Build history of the part. All positions in model axes, mm. Round coordinates to 2 decimals unless told otherwise and drop trailing zeros. Write each loop counter-clockwise with the first axis right and the second up, starting at its lowest first coordinate (ties: lowest second). Pieces come first, ordered by that corner, then holes. Notation, with made-up numbers: (10.25, 39.5) - (14.25, 39.5) arc R22 cw to (14.25, 57.5) - close; hole circle Ø11 at (-8, -35.5). An arc over 180 degrees is marked (long way). Write each question's results on one line, items separated by ' | '.
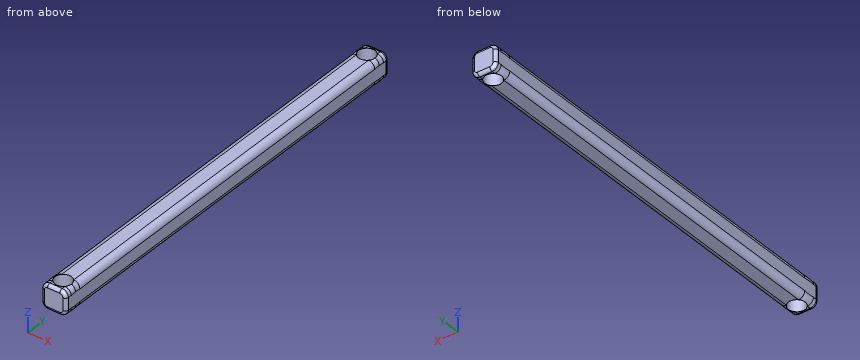
Autodesk Inventor part; units mm, degrees
ref_plane "YZ Plane" through (0, 0, 0) normal (1, 0, 0) x (0, 1, 0)
ref_plane "XZ Plane" through (0, 0, 0) normal (0, 1, 0) x (-1, 0, 0)
ref_plane "XY Plane" through (0, 0, 0) normal (0, 0, 1) x (1, 0, 0)
sketch "Sketch1" plane through (0, 0, 0) normal (0, 1, 0) x (-1, 0, 0)
  line L0 (-3.175, -3.175) -> (3.175, -3.175)
  line L1 (3.175, -3.175) -> (3.175, 3.175)
  line L2 (3.175, 3.175) -> (-3.175, 3.175)
  line L3 (-3.175, 3.175) -> (-3.175, -3.175)
  line L4 (-3.175, -3.175) -> (3.175, 3.175) construction
  line L5 (3.175, -3.175) -> (-3.175, 3.175) construction
  point P0 (0, 0)
  dimension "d0" = 6.35
  dimension "d1" = 6.35
extrude "Extrusion1" add sketch "Sketch1" along normal blind 107.95
sketch "Sketch2" plane through (-3.175, 0, 3.175) normal (0, 0, 1) x (1, 0, 0)
  circle A0 centre (3.175, 3.175) radius 2.159
  line L0 (0, 0) -> (6.35, 0)
  circle A1 centre (3.175, 104.775) radius 2.159
  line L1 (0, 107.95) -> (6.35, 107.95)
  point P0 (3.175, 0)
  dimension "d4" = 4.318
  dimension "d5" = 3.175
  dimension "d6" = 4.318
  dimension "d7" = 3.175
extrude "Extrusion2" cut sketch "Sketch2" against normal blind 101.6
fillet "Fillet1" radius 1.5875 4 edges at (3.175, 53.975, -3.175) (3.175, 53.975, 3.175) (-3.175, 53.975, -3.175) (-3.175, 53.975, 3.175)
fillet "Fillet2" radius 0.7937 16 edges at (2.71, 107.95, -2.71) (0, 107.95, -3.175) (-2.71, 107.95, -2.71) (-3.175, 107.95, 0) (-2.71, 107.95, 2.71) (0, 107.95, 3.175) (2.71, 107.95, 2.71) (3.175, 107.95, 0) (3.175, 0, 0) (2.71, 0, -2.71) (0, 0, -3.175) (-2.71, 0, -2.71) (-3.175, 0, 0) (-2.71, 0, 2.71) (0, 0, 3.175) (2.71, 0, 2.71)
properties part number "30 stop" material "Stainless Steel"
(1) Slice it at C-C, the plane y = 75.5. Write the cut outline in (x, z) (1 decimal).
Worked answers:
outline: (-3.2, -1.6) arc R1.6 ccw to (-1.6, -3.2) - (1.6, -3.2) arc R1.6 ccw to (3.2, -1.6) - (3.2, 1.6) arc R1.6 ccw to (1.6, 3.2) - (-1.6, 3.2) arc R1.6 ccw to (-3.2, 1.6) - close
(2) Drill centre lines: probe 1 along Y at (x, z) = (-1.25, -1.5); probe 2 along Y at (x, z) = (-1, -0.5); probe 3 along X at (y, z) = (70.5, -1.75). Where is each one in solid material? Low to high. Write a range as [from, to].
Worked answers:
probe 1: y = [0, 1.41], [4.94, 103.01], [106.54, 107.95] | probe 2: y = [0, 1.26], [5.09, 102.86], [106.69, 107.95] | probe 3: x = [-3.17, 3.17]
(3) Slice it at B-B, the plane x = 0. Write the cut outline in (y, z) (3 decimals), and give its area (3 significant figures).
Worked answers:
outline: (0, -2.381) arc R0.794 ccw to (0.794, -3.175) - (1.016, -3.175) - (1.016, 3.175) - (0.794, 3.175) arc R0.794 ccw to (0, 2.381) - close; (5.334, -3.175) - (102.616, -3.175) - (102.616, 3.175) - (5.334, 3.175) - close; (106.934, -3.175) - (107.156, -3.175) arc R0.794 ccw to (107.95, -2.381) - (107.95, 2.381) arc R0.794 ccw to (107.156, 3.175) - (106.934, 3.175) - close | area: 630 mm2
(4) Slice it at A-A, the plane z = 0. Write the cut outline in (x, y) (3 decimals).
Worked answers:
outline: (-3.175, 0.794) arc R0.794 ccw to (-2.381, 0) - (2.381, 0) arc R0.794 ccw to (3.175, 0.794) - (3.175, 107.156) arc R0.794 ccw to (2.381, 107.95) - (-2.381, 107.95) arc R0.794 ccw to (-3.175, 107.156) - close; hole circle Ø4.318 at (0, 3.175); hole circle Ø4.318 at (0, 104.775)
(5) Flat gauge pin, fed straight in: pin 1 Ø3 at (y, z) = (33, 2.5) entering from -X (3 decimals). Where does the tip first touch, or does it go through?
Worked answers:
pin 1: stops at x = -3.175
